from build123d import *

# Parameters (mm, degrees)
F1_DEPTH = 38.1
F2_R     = 76.2
F3_R     = 25.4


with BuildPart() as f1:
    # F0 (on Top) → F1 (new body)
    with BuildSketch(Plane.XY):
        Polygon((0, -642.9375), (0, 0), (-1471.7014, 0), (-2475.370745, -1003.669345), (-2475.370745, -1518.108245), (-1832.433245, -1518.108245), (-1832.433245, -1269.982777), (-1205.387968, -642.9375), align=None)
    extrude(amount=F1_DEPTH)

    # F2
    f2_edges = [f1.edges().sort_by_distance(p)[0] for p in [
        (-1832.433245, -1518.108245, 19.05),
    ]]
    fillet(f2_edges, radius=F2_R)

    # F3
    f3_edges = [f1.edges().sort_by_distance(p)[0] for p in [
        (-2475.370745, -1518.108245, 19.05),
    ]]
    fillet(f3_edges, radius=F3_R)


solid = f1.part
Work out the finished part from the listing and answer in its coordinate system (mm). Coordinates: 2 decimals unless noted, no trailing zeros. Loops run counter-clockwise (first coordinate to the right, second up) from the corner with the lowest first, then second, coordinate; pieces in that order, holes last. Notation, with made-up numbers: M 18.5,12.25 L 67.5,12.25 A23 cw 67.5,47.25 Z; hole C 40.25,-1 d1. An arc over 180 degrees is marked long. Answer in a Markdown table with one row per item. Add a question column.
1. Find section A-A, the plane z = 29.5. Write down the section's boundary in (x, y).
2. Find section C-C, the plane x = -782.5. Write down the section's boundary in (y, z), then the cut area to 3 significant figures.
3. Flat-ended cylindrical pins translate along their axes: P1, Ø5, axis at x = -309, y = -509, coming from the -Z side; P2, Ø6, axis at x = -1538.5, y = -980.5, coming from the -Z side; P3, Ø11.5, axis at y = -1358.5, z = 25.5, coming from the +X side; P4, Ø4, axis at y = -967, z = 33.5, coming from the +X side. Find the tip coordinate at first contact, or state that the pin passes through.
4. Find section B-B, the plane y = -1389. Write down the section's boundary in (x, z).
5. Consider L1, parallel to Y at x = -719, z = 3; L2, parallel to X at y = -1378.5, z = 8; L3, parallel to X at y = -1120, z = 4. Determine where each line is inside the solid, lowest interval first.
Reported:
| question | item | result |
|---|---|---|
| 1 | outline | M -2475.37,-1492.71 A25.4 ccw -2449.97,-1518.11 L -1908.63,-1518.11 A76.2 ccw -1832.43,-1441.91 L -1832.43,-1269.98 L -1205.39,-642.94 L 0,-642.94 L 0,0 L -1471.7,0 L -2475.37,-1003.67 Z |
| 2 | outline | M -642.94,0 L 0,0 L 0,38.1 L -642.94,38.1 Z |
| 2 | area | 24,500 mm^2 |
| 3 | P1 | stops at z = 0 |
| 3 | P2 | passes through |
| 3 | P3 | stops at x = -1832.43 |
| 3 | P4 | stops at x = -1527.45 |
| 4 | outline | M -2475.37,0 L -1832.43,0 L -1832.43,38.1 L -2475.37,38.1 Z |
| 5 | L1 | y = -642.94 to 0 |
| 5 | L2 | x = -2475.37 to -1832.43 |
| 5 | L3 | x = -2475.37 to -1682.45 |
